Print and shaded views of the part. All mm, measured from the part's lowest x, y and z. A direction names the side the tool comes from. Coordinates: 2 decimals unless noted, no trailing zeros. Write each question's results on one line, items separated by ' | '.
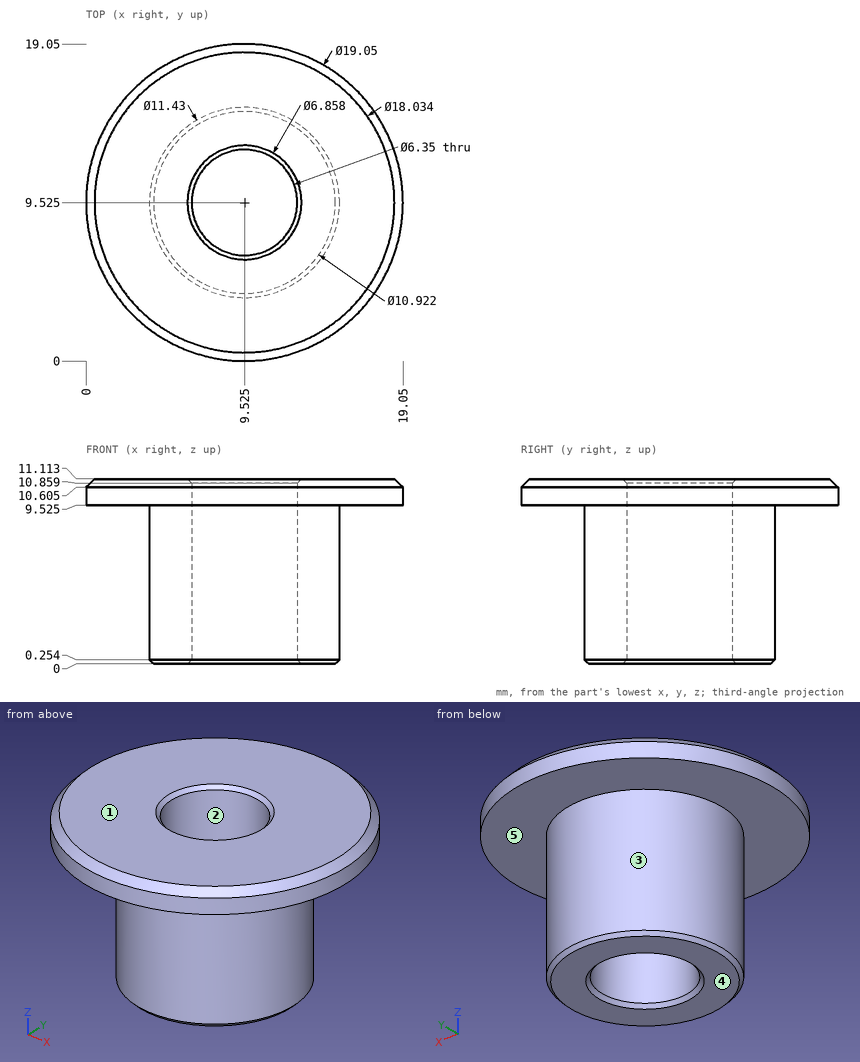
1. Drop flat-ended pins along their axis: pin 1 Ø9.5 at (x, y) = (5.5, 7.5) entering from -Z; pin 2 Ø1 at (x, y) = (16, 14) entering from -Z (1 decimal); pin 3 Ø3 at (x, z) = (7, 4) entering from +Y; pin 4 Ø2 at (y, z) = (3.5, 5.5) entering from -X (1 decimal). Give the stop position or say it passes through.
Solved:
pin 1: stops at z = 0 | pin 2: stops at z = 9.5 | pin 3: stops at y = 15.15 | pin 4: stops at x = 6.8
2. Tool access for the marked faces 4 and 5: list every direction of +Z, -Z, +X, -X, +Y, -Y with a clear straight run to the whole face (end or side of a thin tool).
Solved:
face 4: -Z, +X, -X, +Y, -Y | face 5: -Z
3. Probe line 1 (Z direction, x = 16.5, y = 14.5) (1 decimal); line 2 (Y direction, x = 10.5, z = 8.5) (1 decimal); line 3 (X direction, y = 10, z = 2.75) (1 decimal). List the from-to ranges inside material, lowest first.
Solved:
line 1: z = 9.5 to 11.1 | line 2: y = 3.9 to 6.5, 12.5 to 15.2 | line 3: x = 3.8 to 6.4, 12.7 to 15.2
4. Two-plate mould, pull along X, no slides. Class the marked faces 1, 2 and 3: +X half, -X half, draft (parallel to the pull), parting line (faces both ways), or undercut.
Solved:
face 1: draft | face 2: undercut | face 3: parting line
